CAD build for the part. Positions are in the model's coordinates, mm. Face numbers are marked on the shaded views. A direction names the side the tool comes from. Give positions to 0.01 mm unless a question says otherwise; leave off trailing zeros. Order: outer loops, then holes, each group sorted by start corner. A loop starts at its lowest first (then second) coordinate and runs counter-clockwise, first axis right, second up. Notation, with made-up numbers: M 20,-4.75 L 79,-4.75 A29 ccw 79,34.25 Z; hole C 23.25,-26 d1. An arc over 180 degrees is marked long. Put each result on its own line as item: value. Start each with the question number.
1) Pin check, flat tips, straight feed: pin 1 (6 mm diameter, centred on x = 2, z = -13, fed in from -Y); pin 2 (4.5 mm diameter, centred on x = 12, z = -30, fed in from -Y); pin 3 (6 mm diameter, centred on x = -31.5, z = 20.5, fed in from +Y). Stop position of each tip, or through.
2) Two-plate mould, pull along X, no slides. Class the marked faces 1 and 2: released by +X, released by -X, zero draft, split by the parting line, or undercut.
3) Drill centre lines: line 1 (Z direction, x = 12, y = 2.75); line 2 (Z direction, x = 57.5, y = 1.7); line 3 (Y direction, x = 34, z = 1). Where is each one in solid material? Low to high. Write a range as [from, to].
4) Cut at A-A (z = 0). Give the number of separate pieces and of enclosed holes in the cut face, and give its area (3 significant figures).
5) Tool access for the marked faces 3 and 4: list every direction of +Z, -Z, +X, -X, +Y, -Y with a clear straight run to the whole face (end or side of a thin tool).
6) Cut at B-B (x = 47.5). Write the cut outline in (y, z).
```python
from build123d import *

# Parameters (mm, degrees)
SKETCH_1_W          = 125
SKETCH_1_H          = 68
SKETCH_1_R          = 1.5
SKETCH_1_R_2        = 1.75
SKETCH_1_R_3        = 1.9
EXTRUDE_1_DEPTH     = 2
EXTRUDE_2_DEPTH     = 68
SKETCH_4_W          = 20
SKETCH_4_H          = 2
CUT_EXTRUDE_1_DEPTH = 68
SKETCH_5_R          = 1.8
CUT_EXTRUDE_2_DEPTH = 10


with BuildPart() as part:
    # 草图1 → 凸台-拉伸1 (new body)
    with BuildSketch(Plane(origin=(0, 0, 0), x_dir=(1, 0, 0), z_dir=(0, 1, 0))):
        Rectangle(SKETCH_1_W, SKETCH_1_H)
        with Locations(Location((-57, 0, 0), (0, 0, 270))):
            Circle(SKETCH_1_R, mode=Mode.SUBTRACT)
        with Locations(Location((57, 0, 0), (0, 0, 270))):
            Circle(SKETCH_1_R_2, mode=Mode.SUBTRACT)
        with Locations(Location((57, -29, 0), (0, 0, 270))):
            Circle(SKETCH_1_R_3, mode=Mode.SUBTRACT)
        with Locations(Location((57, 29, 0), (0, 0, 270))):
            Circle(SKETCH_1_R_3, mode=Mode.SUBTRACT)
        with Locations(Location((57, 10.5, 0), (0, 0, 270))):
            Circle(SKETCH_1_R_2, mode=Mode.SUBTRACT)
        with Locations(Location((57, -10.5, 0), (0, 0, 270))):
            Circle(SKETCH_1_R_2, mode=Mode.SUBTRACT)
        with Locations(Location((-57, 10.5, 0), (0, 0, 270))):
            Circle(SKETCH_1_R_2, mode=Mode.SUBTRACT)
        with Locations(Location((-57, -10.5, 0), (0, 0, 270))):
            Circle(SKETCH_1_R_2, mode=Mode.SUBTRACT)
        with Locations(Location((-57, 29, 0), (0, 0, 270))):
            Circle(SKETCH_1_R_3, mode=Mode.SUBTRACT)
        with Locations(Location((-57, -29, 0), (0, 0, 270))):
            Circle(SKETCH_1_R_3, mode=Mode.SUBTRACT)
    extrude(amount=EXTRUDE_1_DEPTH)

    # 草图3 → 凸台-拉伸2 (add)
    with BuildSketch(Plane.XY.offset(34)):
        with BuildLine():
            Line((-40, 0), (40, 0))
            add(Edge.make_bspline(
                [(-40, 0), (-26.931059471, 3.210455026), (0, 4.789544974), (26.931059471, 3.210455026), (40, 0)],
                knots=[0, 0, 0, 0, 0.5, 1, 1, 1, 1], degree=3))
        make_face()
    extrude(amount=-EXTRUDE_2_DEPTH)

    # 草图4 → 切除-拉伸1 (cut)
    with BuildSketch(Plane.XY.offset(34)):
        with Locations((0, 1)):
            Rectangle(SKETCH_4_W, SKETCH_4_H)
        with BuildLine():
            Line((-10, 0), (-10, 2))
            add(Edge.make_bspline(
                [(-20, 0), (-15.076813979, 1.384660804), (-10, 2)],
                knots=[0, 0, 0, 1, 1, 1], degree=2))
            Line((-20, 0), (-10, 0))
        make_face()
        with BuildLine():
            add(Edge.make_bspline(
                [(10, 2), (15.076813979, 1.384660804), (20, 0)],
                knots=[0, 0, 0, 1, 1, 1], degree=2))
            Line((10, 2), (10, 0))
            Line((10, 0), (20, 0))
        make_face()
    extrude(amount=-CUT_EXTRUDE_1_DEPTH, mode=Mode.SUBTRACT)

    # 草图5 → 切除-拉伸2 (cut)
    with BuildSketch(Plane(origin=(0, 0, 0), x_dir=(1, 0, 0), z_dir=(0, 1, 0))):
        with Locations(Location((-24.5, 30, 0), (0, 0, 90))):
            Circle(SKETCH_5_R)
        with Locations(Location((-12, 30, 0), (0, 0, 90))):
            Circle(SKETCH_5_R)
        with Locations(Location((12, 30, 0), (0, 0, 90))):
            Circle(SKETCH_5_R)
        with Locations(Location((24.5, 30, 0), (0, 0, 90))):
            Circle(SKETCH_5_R)
    extrude(amount=CUT_EXTRUDE_2_DEPTH, mode=Mode.SUBTRACT)


solid = part.part
```
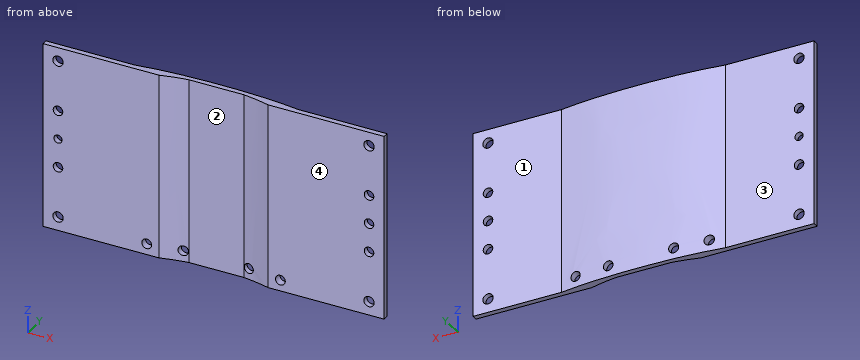
Solution:
1. pin 1: y = 2
1. pin 2: y = 1.35
1. pin 3: y = 2.23
2. face 1: zero draft
2. face 2: undercut
3. line 1: [-34, -31.8], [-28.2, 34]
3. line 2: [-34, -30.83], [-27.17, -12.18], [-8.82, -1.68], [1.68, 8.82], [12.18, 27.17], [30.83, 34]
3. line 3: [0, 2]
4. separate pieces: 3
4. enclosed holes: 0
4. area: 258 mm²
5. face 3: +Z, -Z, -X, +Y
5. face 4: +Z, -Z, +X, -X, -Y
6. outline: M 0,-34 L 2,-34 L 2,34 L 0,34 Z
